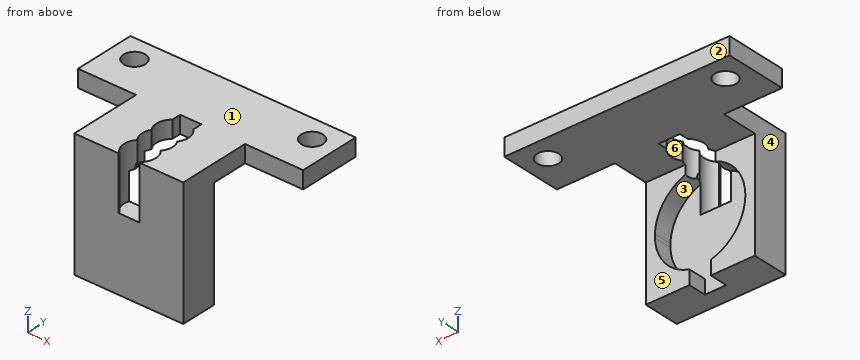
```python
from build123d import *

# Parameters (mm, degrees)
SKETCH_1_W                = 70
SKETCH_1_H                = 43
EXTRUDE_1_DEPTH           = 10
SKETCH_8_W                = 24.88
SKETCH_8_H                = 5
CUT_EXTRUDE_4_DEPTH       = 57.338264084
EXTRUDE_1_2_DEPTH         = 5
EXTRUDE_1_2_DEPTH_BACK    = 2
SKETCH_11_R               = 20.45
SKETCH_11_R_2             = 12.45
CUT_EXTRUDE_6_DEPTH       = 5
CUT_EXTRUDE_7_DEPTH       = 5
SKETCH_16_W               = 5.88
SKETCH_16_H               = 11
CUT_EXTRUDE_8_DEPTH       = 5
SKETCH_17_W               = 5.88
SKETCH_17_H               = 8.352111755
CUT_EXTRUDE_9_DEPTH       = 5
CUT_EXTRUDE_10_DEPTH      = 5
CUT_EXTRUDE_11_DEPTH      = 5
SKETCH_21_R               = 3
CUT_EXTRUDE_12_DEPTH      = 43.275879648
SKETCH_22_R               = 3
CUT_EXTRUDE_13_DEPTH      = 43.275879648
SKETCH_24_R               = 3.51
CUT_EXTRUDE_15_DEPTH      = 7
SKETCH_25_W               = 22.5
SKETCH_25_H               = 10
EXTRUDE_2_DEPTH           = 5
SKETCH_26_W               = 22.62
SKETCH_26_H               = 10
EXTRUDE_3_DEPTH           = 5
SKETCH_28_W               = 5.88
SKETCH_28_H               = 7.531424881
CUT_EXTRUDE_16_DEPTH      = 5
CUT_EXTRUDE_2_DEPTH       = 45
CUT_EXTRUDE_2_DEPTH_BACK  = 31
SKETCH_32_W               = 110
SKETCH_32_H               = 112
SKETCH_32_W_2             = 30
SKETCH_32_H_2             = 32
SKETCH_33_W               = 12
SKETCH_33_H               = 10
SKETCH_33_W_2             = 12.12
EXTRUDE_5_DEPTH           = 3
SKETCH_40_W               = 12
SKETCH_40_H               = 4.777354505
EXTRUDE_7_DEPTH           = 10
SKETCH_41_W               = 12.12
SKETCH_41_H               = 4.777354505
EXTRUDE_8_DEPTH           = 10
CUT_EXTRUDE_17_DEPTH      = 10
CUT_EXTRUDE_17_DEPTH_BACK = 10
SKETCH_42_R               = 4.209320402
SKETCH_53_W               = 4.777354505
SKETCH_53_H               = 10
EXTRUDE_9_DEPTH           = 11
SKETCH_56_W               = 4.777354505
SKETCH_56_H               = 20
EXTRUDE_10_DEPTH          = 11
SKETCH_57_W               = 4.777354505
SKETCH_57_H               = 10
CUT_EXTRUDE_18_DEPTH      = 11
SKETCH_58_W               = 4.777354505
SKETCH_58_H               = 10
EXTRUDE_11_DEPTH          = 5
SKETCH_59_W               = 4.777354505
SKETCH_59_H               = 10
EXTRUDE_12_DEPTH          = 5
SKETCH_60_W               = 62
SKETCH_60_H               = 4.777354505
EXTRUDE_13_DEPTH          = 10
SKETCH_61_W               = 5.88
SKETCH_61_H               = 5
CUT_EXTRUDE_19_DEPTH      = 10
SKETCH_69_W               = 4.777354505
SKETCH_69_H               = 10
EXTRUDE_14_DEPTH          = 16
SKETCH_70_W               = 4.777354505
SKETCH_70_H               = 10
EXTRUDE_15_DEPTH          = 16
SKETCH_83_W               = 62
SKETCH_83_H               = 4.777354505
EXTRUDE_16_DEPTH          = 29
SKETCH_86_R               = 3
CUT_EXTRUDE_20_DEPTH      = 76.279479276
SKETCH_85_R               = 3
CUT_EXTRUDE_21_DEPTH      = 76.279479276
SKETCH_87_W               = 62
SKETCH_87_H               = 22
CUT_EXTRUDE_22_DEPTH      = 76.279479276
SKETCH_90_W               = 16.042506896
SKETCH_90_H               = 20
SKETCH_90_W_2             = 16.042536038
CUT_EXTRUDE_23_DEPTH      = 10
SKETCH_91_R               = 4.404741758
CUT_EXTRUDE_24_DEPTH      = 10
SKETCH_92_R               = 4.366810658
CUT_EXTRUDE_25_DEPTH      = 53.335030246


with BuildPart() as part:
    # 草圖1 → Extrude 1 (new body)
    with BuildSketch(Plane(origin=(0, 0, 0), x_dir=(1, 0, 0), z_dir=(0, 1, 0))):
        Rectangle(SKETCH_1_W, SKETCH_1_H)
    extrude(amount=EXTRUDE_1_DEPTH)

    # 草圖8 → 除料-伸長4 (cut, through all)
    with BuildSketch(Plane.XY.offset(21.5)):
        with Locations((0.06, 7.5)):
            Rectangle(SKETCH_8_W, SKETCH_8_H)
    extrude(amount=-CUT_EXTRUDE_4_DEPTH, mode=Mode.SUBTRACT)

    # 草圖11 → Extrude 1 2 (add, two sides: drawn at the far end of the back side and taken through both)
    with BuildSketch(Plane(origin=(0, 5, 0), x_dir=(1, 0, 0), z_dir=(0, 1, 0)).offset(-EXTRUDE_1_2_DEPTH_BACK)):
        with Locations((0.06, 0)):
            Circle(SKETCH_11_R)
        with Locations((0.06, 0)):
            Circle(SKETCH_11_R_2, mode=Mode.SUBTRACT)
    extrude(amount=EXTRUDE_1_2_DEPTH + EXTRUDE_1_2_DEPTH_BACK)

    # 草圖14 → 除料-伸長6 (cut)
    with BuildSketch(Plane(origin=(0, 5, 0), x_dir=(1, 0, 0), z_dir=(0, 1, 0))):
        Polygon((0.06, -20.45), (12.5, -20.45), (12.5, -21.5), (-12.38, -21.5), (-12.38, -20.45), align=None)
    extrude(amount=-CUT_EXTRUDE_6_DEPTH, mode=Mode.SUBTRACT)

    # 草圖15 → 除料-伸長7 (cut)
    with BuildSketch(Plane(origin=(0, 5, 0), x_dir=(1, 0, 0), z_dir=(0, 1, 0))):
        Polygon((0.06, 20.45), (12.5, 20.45), (12.5, 21.5), (-12.38, 21.5), (-12.38, 20.45), align=None)
    extrude(amount=-CUT_EXTRUDE_7_DEPTH, mode=Mode.SUBTRACT)

    # 草圖16 → 除料-伸長8 (cut)
    with BuildSketch(Plane(origin=(0, 10, 0), x_dir=(1, 0, 0), z_dir=(0, 1, 0))):
        with Locations((0.06, 17.597888245)):
            Rectangle(SKETCH_16_W, SKETCH_16_H)
    extrude(amount=-CUT_EXTRUDE_8_DEPTH, mode=Mode.SUBTRACT)

    # 草圖17 → 除料-伸長9 (cut)
    with BuildSketch(Plane(origin=(0, 10, 0), x_dir=(1, 0, 0), z_dir=(0, 1, 0))):
        with Locations((0.06, -16.273944123)):
            Rectangle(SKETCH_17_W, SKETCH_17_H)
    extrude(amount=-CUT_EXTRUDE_9_DEPTH, mode=Mode.SUBTRACT)

    # 草圖19 → 除料-伸長10 (cut)
    with BuildSketch(Plane(origin=(0, 5, 0), x_dir=(1, 0, 0), z_dir=(0, 1, 0))):
        Polygon((-2.88, 20.237561612), (-2.88, 20.45), (2.98755849, 20.45), (3, 20.237561612), align=None)
    extrude(amount=-CUT_EXTRUDE_10_DEPTH, mode=Mode.SUBTRACT)

    # 草圖20 → 除料-伸長11 (cut)
    with BuildSketch(Plane(origin=(0, 5, 0), x_dir=(1, 0, 0), z_dir=(0, 1, 0))):
        Polygon((3, -20.237561612), (3, -20.45), (-2.887827835, -20.45), (-2.88, -20.237561612), align=None)
    extrude(amount=-CUT_EXTRUDE_11_DEPTH, mode=Mode.SUBTRACT)

    # 草圖21 → 除料-伸長12 (cut, through all)
    with BuildSketch(Plane(origin=(0, 10, 0), x_dir=(1, 0, 0), z_dir=(0, 1, 0))):
        with Locations(Location((-25, 11.5, 0), (0, 0, 270))):
            Circle(SKETCH_21_R)
    extrude(amount=-CUT_EXTRUDE_12_DEPTH, mode=Mode.SUBTRACT)

    # 草圖22 → 除料-伸長13 (cut, through all)
    with BuildSketch(Plane(origin=(0, 10, 0), x_dir=(1, 0, 0), z_dir=(0, 1, 0))):
        with Locations(Location((25, 11.5, 0), (0, 0, 270))):
            Circle(SKETCH_22_R)
    extrude(amount=-CUT_EXTRUDE_13_DEPTH, mode=Mode.SUBTRACT)

    # 草圖24 → 除料-伸長15 (cut)
    with BuildSketch(Plane(origin=(0, 5, 0), x_dir=(1, 0, 0), z_dir=(0, 1, 0))):
        with Locations((0, -12.216230782)):
            Circle(SKETCH_24_R)
    extrude(amount=CUT_EXTRUDE_15_DEPTH, mode=Mode.SUBTRACT)

    # 草圖25 → 填料-伸長2 (add)
    with BuildSketch(Plane.XY.offset(21.5)):
        with Locations((23.75, 5)):
            Rectangle(SKETCH_25_W, SKETCH_25_H)
    extrude(amount=EXTRUDE_2_DEPTH)

    # 草圖26 → 填料-伸長3 (add)
    with BuildSketch(Plane.XY.offset(21.5)):
        with Locations((-23.69, 5)):
            Rectangle(SKETCH_26_W, SKETCH_26_H)
    extrude(amount=EXTRUDE_3_DEPTH)

    # 草圖28 → 除料-伸長16 (cut)
    with BuildSketch(Plane(origin=(0, 5, 0), x_dir=(1, 0, 0), z_dir=(0, 1, 0))):
        with Locations((0.06, -17.988357936)):
            Rectangle(SKETCH_28_W, SKETCH_28_H)
    extrude(amount=-CUT_EXTRUDE_16_DEPTH, mode=Mode.SUBTRACT)

    # 草圖32 → 除料-伸長-薄件2 (cut, two sides: drawn at the far end of the back side and taken through both)
    with BuildSketch(Plane(origin=(0, 5, 0), x_dir=(1, 0, 0), z_dir=(0, 1, 0)).offset(-CUT_EXTRUDE_2_DEPTH_BACK)):
        Rectangle(SKETCH_32_W, SKETCH_32_H)
        Rectangle(SKETCH_32_W_2, SKETCH_32_H_2, mode=Mode.SUBTRACT)
    extrude(amount=CUT_EXTRUDE_2_DEPTH + CUT_EXTRUDE_2_DEPTH_BACK, mode=Mode.SUBTRACT)

    # 草圖33 → 填料-伸長5 (add)
    with BuildSketch(Plane.XY.offset(16)):
        with Locations((9, 5)):
            Rectangle(SKETCH_33_W, SKETCH_33_H)
        with Locations((-8.94, 5)):
            Rectangle(SKETCH_33_W_2, SKETCH_33_H)
    extrude(amount=EXTRUDE_5_DEPTH)

    # 草圖40 → 填料-伸長7 (add)
    with BuildSketch(Plane(origin=(0, 10, 0), x_dir=(1, 0, 0), z_dir=(0, 1, 0))):
        with Locations((9, -16.611322748)):
            Rectangle(SKETCH_40_W, SKETCH_40_H)
    extrude(amount=EXTRUDE_7_DEPTH)

    # 草圖41 → 填料-伸長8 (add)
    with BuildSketch(Plane(origin=(0, 10, 0), x_dir=(1, 0, 0), z_dir=(0, 1, 0))):
        with Locations((-8.94, -16.611322748)):
            Rectangle(SKETCH_41_W, SKETCH_41_H)
    extrude(amount=EXTRUDE_8_DEPTH)

    # 草圖42 → 除料-伸長17 (cut, two sides: drawn at the far end of the back side and taken through both)
    with BuildSketch(Plane.XY.offset(14.222645495).offset(-CUT_EXTRUDE_17_DEPTH_BACK)):
        with Locations((0, 9.264740645)):
            Circle(SKETCH_42_R)
    extrude(amount=CUT_EXTRUDE_17_DEPTH + CUT_EXTRUDE_17_DEPTH_BACK, mode=Mode.SUBTRACT)

    # 草圖53 → 填料-伸長9 (add)
    with BuildSketch(Plane.ZY.offset(15)):
        with Locations((16.611322748, 15)):
            Rectangle(SKETCH_53_W, SKETCH_53_H)
    extrude(amount=EXTRUDE_9_DEPTH)

    # 草圖56 → 填料-伸長10 (add)
    with BuildSketch(Plane(origin=(15, 0, 0), x_dir=(0, 0, -1), z_dir=(1, 0, 0))):
        with Locations((-16.611322748, 10)):
            Rectangle(SKETCH_56_W, SKETCH_56_H)
    extrude(amount=EXTRUDE_10_DEPTH)

    # 草圖57 → 除料-伸長18 (cut)
    with BuildSketch(Plane(origin=(26, 0, 0), x_dir=(0, 0, -1), z_dir=(1, 0, 0))):
        with Locations((-16.611322748, 5)):
            Rectangle(SKETCH_57_W, SKETCH_57_H)
    extrude(amount=-CUT_EXTRUDE_18_DEPTH, mode=Mode.SUBTRACT)

    # 草圖58 → 填料-伸長11 (add)
    with BuildSketch(Plane(origin=(26, 0, 0), x_dir=(0, 0, -1), z_dir=(1, 0, 0))):
        with Locations((-16.611322748, 15)):
            Rectangle(SKETCH_58_W, SKETCH_58_H)
    extrude(amount=EXTRUDE_11_DEPTH)

    # 草圖59 → 填料-伸長12 (add)
    with BuildSketch(Plane.ZY.offset(26)):
        with Locations((16.611322748, 15)):
            Rectangle(SKETCH_59_W, SKETCH_59_H)
    extrude(amount=EXTRUDE_12_DEPTH)

    # 草圖60 → 填料-伸長13 (add)
    with BuildSketch(Plane(origin=(0, 20, 0), x_dir=(1, 0, 0), z_dir=(0, 1, 0))):
        with Locations((0, -16.611322748)):
            Rectangle(SKETCH_60_W, SKETCH_60_H)
    extrude(amount=EXTRUDE_13_DEPTH)

    # 草圖61 → 除料-伸長19 (cut)
    with BuildSketch(Plane.XY.offset(14.222645495)):
        with Locations((0.06, 2.5)):
            Rectangle(SKETCH_61_W, SKETCH_61_H)
    extrude(amount=-CUT_EXTRUDE_19_DEPTH, mode=Mode.SUBTRACT)

    # 草圖69 → 填料-伸長14 (add)
    with BuildSketch(Plane(origin=(15, 0, 0), x_dir=(0, 0, -1), z_dir=(1, 0, 0))):
        with Locations((-16.611322748, 5)):
            Rectangle(SKETCH_69_W, SKETCH_69_H)
    extrude(amount=EXTRUDE_14_DEPTH)

    # 草圖70 → 填料-伸長15 (add)
    with BuildSketch(Plane.ZY.offset(15)):
        with Locations((16.611322748, 5)):
            Rectangle(SKETCH_70_W, SKETCH_70_H)
    extrude(amount=EXTRUDE_15_DEPTH)

    # 草圖83 → 填料-伸長16 (add)
    with BuildSketch(Plane(origin=(0, 30, 0), x_dir=(1, 0, 0), z_dir=(0, 1, 0))):
        with Locations((0, -16.611322748)):
            Rectangle(SKETCH_83_W, SKETCH_83_H)
    extrude(amount=EXTRUDE_16_DEPTH)

    # 草圖86 → 除料-伸長20 (cut, through all)
    with BuildSketch(Plane.XY.offset(19)):
        with Locations((-24.38, 30.52)):
            Circle(SKETCH_86_R)
    extrude(amount=-CUT_EXTRUDE_20_DEPTH, mode=Mode.SUBTRACT)

    # 草圖85 → 除料-伸長21 (cut, through all)
    with BuildSketch(Plane.XY.offset(19)):
        with Locations((24.5, 30.52)):
            Circle(SKETCH_85_R)
    extrude(amount=-CUT_EXTRUDE_21_DEPTH, mode=Mode.SUBTRACT)

    # 草圖87 → 除料-伸長22 (cut, through all)
    with BuildSketch(Plane.XY.offset(19)):
        with Locations((0, 48)):
            Rectangle(SKETCH_87_W, SKETCH_87_H)
    extrude(amount=-CUT_EXTRUDE_22_DEPTH, mode=Mode.SUBTRACT)

    # 草圖90 → 除料-伸長23 (cut)
    with BuildSketch(Plane(origin=(0, 0, 14.222645495), x_dir=(-1, 0, 0), z_dir=(0, 0, -1))):
        with Locations((23.021253448, 10)):
            Rectangle(SKETCH_90_W, SKETCH_90_H)
        with Locations((-23.021268019, 10)):
            Rectangle(SKETCH_90_W_2, SKETCH_90_H)
    extrude(amount=-CUT_EXTRUDE_23_DEPTH, mode=Mode.SUBTRACT)

    # 草圖91 → 除料-伸長24 (cut)
    with BuildSketch(Plane.XY.offset(19)):
        with Locations((0, 14.133466634)):
            Circle(SKETCH_91_R)
    extrude(amount=-CUT_EXTRUDE_24_DEPTH, mode=Mode.SUBTRACT)

    # 草圖92 → 除料-伸長25 (cut, through all)
    with BuildSketch(Plane.XY.offset(4.222645495)):
        with Locations((0, 3.605723159)):
            Circle(SKETCH_92_R)
    extrude(amount=CUT_EXTRUDE_25_DEPTH, mode=Mode.SUBTRACT)


solid = part.part
```
Here's how the part is built. I have some questions about the finished solid (model axes, mm). Face numbers are marked on the shaded views. A direction names the side the tool comes from. Coordinates: 2 decimals unless noted, no trailing zeros. Order: outer loops, then holes, each group sorted by start corner. A loop starts at its lowest first (then second) coordinate and runs counter-clockwise, first axis right, second up. Notation, with made-up numbers: M -24,69 L 28,69 A26 cw 28,93 Z; hole C 72,23.5 d4. An arc over 180 degrees is marked long. Answer as a JSON object with one key per item and string values. Group by question number.
(1) Suppose I cut it at D-D, the plane x = 24.5. Please give me the cut outline in (y, z).
(2) Suppose I cut it at B-B, the plane y = 30.52. Please give me the cut outline in (x, z).
(3) I need wall thicknesses on probe 1 along X at (y, z) = (30, 15); probe 2 along Y at (x, z) = (-6, 5); probe 3 along Y at (x, z) = (6, -13.5). Which ranges of each line are inside material? Lowest first, please.
(4) For pin 1 (1.3 mm diameter, centred on y = 19, z = 16, fed in from -X); pin 2 (13 mm diameter, centred on x = 9.5, z = 3.5, fed in from +Y); pin 3 (5.5 mm diameter, centred on x = -26.5, z = 16, fed in from -Y), each with a flat end and sliding along its axis, tell me the tip position at first contact or that it passes through.
(5) Suppose I cut it at A-A, the plane x = 0. Please give me the cut outline in (y, z), then the cut area to 3 significant figures.
(6) Which directions (+Z, -Z, +X, -X, +Y, -Y) give clear straight access to the entire face, cutting with the end or side of a thin tool? Please do the marked faces 4, 5 and 6.
(7) If we mould it in two halves opening along Z, with no side actions, what happens to the marked faces 1, 2 and 3? For each: released by +Z, released by -Z, zero draft, split by the parting line, or undercut.
(8) Suppose I cut it at C-C, the plane z = -13.5. Please give me the cut outline in (x, y).
Values found:
{
 "1": {"outline": "M 20,14.22 L 27.52,14.22 L 27.52,19 L 20,19 Z; M 33.52,14.22 L 37,14.22 L 37,19 L 33.52,19 Z"},
 "2": {"outline": "M -31,14.22 L -27.38,14.22 L -27.38,19 L -31,19 Z; M -21.38,14.22 L 21.5,14.22 L 21.5,19 L -21.38,19 Z; M 27.5,14.22 L 31,14.22 L 31,19 L 27.5,19 Z"},
 "3": {"probe 1": "x = -31 to -27.33, -21.43 to 21.55, 27.45 to 31", "probe 2": "y = 0 to 5", "probe 3": "y = 0 to 10"},
 "4": {"pin 1": "stops at x = -15", "pin 2": "stops at y = 10", "pin 3": "stops at y = 20"},
 "5": {"outline": "M 0,-16 L 5,-16 L 5,4.22 L 0,4.22 Z; M 20,14.22 L 37,14.22 L 37,19 L 20,19 Z", "area": "182 mm^2"},
 "6": {"face 4": "+Z, -Z, -X, -Y", "face 5": "-Z, +X, -X, +Y", "face 6": "+Z, -Z"},
 "7": {"face 1": "released by +Z", "face 2": "zero draft", "face 3": "undercut"},
 "8": {"outline": "M -15,0 L 15,0 L 15,10 L 3,10 L 3,5 L -2.88,5 L -2.88,10 L -15,10 Z"}
}
